```python
from build123d import *

# Parameters (mm, degrees)
BOSS_EXTRUDE1_DEPTH = 19.05


with BuildPart() as part:
    # Sketch1 → Revolve1 (revolve)
    with BuildSketch(Plane.XY, mode=Mode.PRIVATE) as revolve1_sk:
        Polygon((-4, -19.7), (0, -19.7), (0, 19.7), (-4, 19.7), (-4, 12.7), (-7.9375, 12.7), (-7.9375, 9.525), (-12.7, 9.525), (-12.7, -9.525), (-7.9375, -9.525), (-7.9375, -12.7), (-4, -12.7), align=None)
    revolve(revolve1_sk.sketch.rotate(Axis((0, 0, 0), (0, 1, 0)), 180), axis=Axis((0, 0, 0), (0, 1, 0)))

    # Sketch2 → Boss-Extrude1 (add)
    with BuildSketch(Plane(origin=(0, 9.525, 0), x_dir=(1, 0, 0), z_dir=(0, 1, 0))):
        Polygon((12.7, 0), (23.672555951, 9.207067652), (12.7, 22.283650626), (-12.7, 22.283650626), (-12.7, 0), align=None)
    extrude(amount=-BOSS_EXTRUDE1_DEPTH)


solid = part.part
```
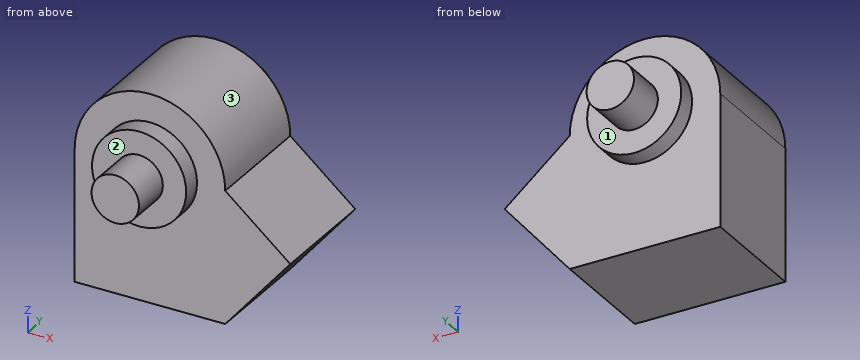
Input: part model. Units: mm. Frame: model coordinates. Face numbers are marked on the shaded views. A direction names the side the tool comes from. Give positions to 0.01 mm unless a question says otherwise; leave off trailing zeros. Order: outer loops, then holes, each group sorted by start corner. A loop starts at its lowest first (then second) coordinate and runs counter-clockwise, first axis right, second up. Notation, with made-up numbers: M 18.25,2.25 L 67.25,2.25 A10 cw 67.25,12.25 Z; hole C 51.25,-16.75 d3. An arc over 180 degrees is marked long. Return JSON: item names as keys, results as strings.
Item 1: First-contact query: P1, Ø3, axis at y = 1.5, z = -14.5, coming from the +X side; P2, Ø6, axis at y = 15.5, z = -18.5, coming from the +X side; P3, Ø17.5, axis at x = 8.5, z = -10, coming from the +Y side; P4, Ø5, axis at x = 6, y = -5.5, coming from the +Z side. Flat tips, straight axial feed; report the tip coordinate or a pass-through.
Solutions:
{"P1": "x = 20.49", "P2": "through", "P3": "y = 12.7", "P4": "z = 12.21"}
Item 2: Cut plane B-B (z = -5). Return loops of the section in (x, y) (3 decimals), then the cut area to 3 significant figures.
Solutions:
{"outline": "M -12.7,-9.525 L -6.165,-9.525 L -6.165,-12.7 L 6.165,-12.7 L 6.165,-9.525 L 18.659,-9.525 L 18.659,9.525 L 6.165,9.525 L 6.165,12.7 L -6.165,12.7 L -6.165,9.525 L -12.7,9.525 Z", "area": "676 mm^2"}
Item 3: Ray query, probe 1 along Y at (x, z) = (13.5, -12) (3 decimals); probe 2 along Z at (x, y) = (0.5, -6); probe 3 along X at (y, z) = (6.5, -4.5). Return the intervals inside material, ascending.
Solutions:
{"probe 1": "-9.525 to 9.525", "probe 2": "-22.28 to 12.69", "probe 3": "-12.7 to 18.06"}
Item 4: Cut plane A-A (x = 0). Return loops of the section in (y, z) (1 decimal).
Solutions:
{"outline": "M -19.7,-4 L -12.7,-4 L -12.7,-7.9 L -9.5,-7.9 L -9.5,-22.3 L 9.5,-22.3 L 9.5,-7.9 L 12.7,-7.9 L 12.7,-4 L 19.7,-4 L 19.7,4 L 12.7,4 L 12.7,7.9 L 9.5,7.9 L 9.5,12.7 L -9.5,12.7 L -9.5,7.9 L -12.7,7.9 L -12.7,4 L -19.7,4 Z"}
Item 5: Cut plane C-C (y = -9). Return loops of the section in (x, z).
Solutions:
{"outline": "M -12.7,-22.28 L 12.7,-22.28 L 23.67,-9.21 L 12.7,0 A12.7 ccw -12.7,0 Z"}
Item 6: Cut plane D-D (z = 5.5). Return loops of the section in (x, y) (3 decimals), then the cut area to 3 significant figures.
Solutions:
{"outline": "M -11.447,-9.525 L -5.723,-9.525 L -5.723,-12.7 L 5.723,-12.7 L 5.723,-9.525 L 11.447,-9.525 L 11.447,9.525 L 5.723,9.525 L 5.723,12.7 L -5.723,12.7 L -5.723,9.525 L -11.447,9.525 Z", "area": "509 mm^2"}
Item 7: Access query for the marked faces 1, 2 and 3. Directions: +Z, -Z, +X, -X, +Y, -Y. A direction counts if a zero-diameter tool reaches every point of the face in a straight line with its end or side. Return the directions, or none.
Solutions:
{"face 1": "+Y", "face 2": "-Y", "face 3": "+Z, +Y, -Y"}
